Build history of the part. All positions in model axes, mm. Face numbers are marked on the shaded views. A direction names the side the tool comes from. Coordinates: 2 decimals unless noted, no trailing zeros. Order: outer loops, then holes, each group sorted by start corner. A loop starts at its lowest first (then second) coordinate and runs counter-clockwise, first axis right, second up. Notation, with made-up numbers: (55.25, 45) - (89.25, 45) arc R28 cw to (89.25, 67) - close; hole circle Ø9 at (6.5, -12). An arc over 180 degrees is marked (long way). Return JSON: item names as keys, results as strings.
Autodesk Inventor part; units mm, degrees
ref_plane "YZ Plane" through (0, 0, 0) normal (1, 0, 0) x (0, 1, 0)
ref_plane "XZ Plane" through (0, 0, 0) normal (0, 1, 0) x (-1, 0, 0)
ref_plane "XY Plane" through (0, 0, 0) normal (0, 0, 1) x (1, 0, 0)
sketch "Sketch2" plane through (0, 0, 0) normal (0, 1, 0) x (-1, 0, 0)
  line L0 (0, 0) -> (0, -39.2)
  line L1 (0, -39.2) -> (-69.3, -39.2)
  line L2 (-69.3, -39.2) -> (-69.3, 0)
  line L3 (-69.3, 0) -> (0, 0)
  dimension "d0" = 39.2
  dimension "d1" = 69.3
extrude "Extrusion1" add sketch "Sketch2" against normal blind 5
sketch "Sketch3" plane through (0, -5, 0) normal (0, -1, 0) x (1, 0, 0)
  line L0 (0, 0) -> (0, -39.2)
  line L1 (0, -39.2) -> (0, -34.2)
  line L2 (0, -34.2) -> (69.3, -34.2)
  line L3 (69.3, -39.2) -> (69.3, 0)
  line L4 (69.3, -39.2) -> (69.3, -34.2)
  line L5 (0, -39.2) -> (69.3, -39.2)
  dimension "d4" = 5
extrude "Extrusion2" add sketch "Sketch3" along normal blind 20
sketch "Sketch4" plane through (0, -5, -34.2) normal (0, 0, 1) x (1, 0, 0)
  line L0 (0, 5) -> (0, -20)
  line L1 (0, -20) -> (0, -18)
  line L2 (0, -18) -> (69.3, -18)
  line L3 (69.3, 5) -> (69.3, -20)
  line L4 (69.3, -20) -> (69.3, -18)
  line L5 (0, -20) -> (69.3, -20)
  line L6 (0, -20) -> (69.3, -20)
  dimension "d7" = 2
extrude "Extrusion3" add sketch "Sketch4" along normal blind 5
sketch "Sketch5" plane through (69.3, 0, 0) normal (1, 0, 0) x (0, 0, -1)
  line L0 (39.2, -25) -> (29.2, -25)
  line L1 (29.2, -25) -> (29.2, 0)
  line L2 (39.2, 0) -> (0, 0)
  line L3 (29.2, 0) -> (39.2, 0)
  line L4 (39.2, 0) -> (39.2, -25)
  line L5 (39.2, -25) -> (29.2, -25)
extrude "Extrusion4" add sketch "Sketch5" along normal blind 5
sketch "Sketch6" plane through (69.3, -5, 0) normal (1, 0, 0) x (0, 0, -1)
  line L0 (0, 5) -> (0, 0)
  line L1 (29.2, 0) -> (29.2, 5)
  line L2 (0, 5) -> (29.2, 5)
  line L3 (29.2, 5) -> (29.2, 0)
  line L4 (0, 0) -> (34.2, 0)
  line L5 (29.2, 0) -> (0, 0)
  line L6 (0, 0) -> (0, 5)
extrude "Extrusion5" add sketch "Sketch6" along normal blind 5
sketch "Sketch7" plane through (0, -5, -29.2) normal (0, 0, 1) x (1, 0, 0)
  line L0 (0, -20) -> (74.3, -20)
  line L1 (74.3, -20) -> (74.3, 0)
  line L2 (74.3, 0) -> (69.3, 0)
  line L3 (74.3, 0) -> (69.3, 0)
  line L4 (69.3, 0) -> (69.3, -18)
  line L5 (69.3, 0) -> (69.3, -20)
  line L6 (74.3, -20) -> (69.3, -20)
  point P0 (0, 5)
extrude "Extrusion6" add sketch "Sketch7" along normal up to surface (29.2 mm away)
sketch "Sketch8" plane through (0, 0, -39.2) normal (-1, 0, 0) x (0, 0, 1)
  line L0 (10, -25) -> (39.2, -25)
  line L1 (10, -25) -> (10, 0)
  line L2 (0, 0) -> (39.2, 0)
  line L3 (0, 0) -> (10, 0)
  line L4 (0, 0) -> (0, -25)
  line L5 (0, -25) -> (10, -25)
extrude "Extrusion7" add sketch "Sketch8" along normal blind 5
sketch "Sketch9" plane through (0, -5, 0) normal (-1, 0, 0) x (0, 0, 1)
  line L0 (-29.2, 5) -> (0, 5)
  line L1 (0, 5) -> (-29.2, 5)
  line L2 (-39.2, -20) -> (-29.2, -20)
  line L3 (-29.2, 5) -> (-29.2, -20)
  line L4 (0, 5) -> (0, -20)
  line L5 (-29.2, -20) -> (0, -20)
  line L6 (0, -20) -> (0, 5)
extrude "Extrusion8" add sketch "Sketch9" along normal blind 5
sketch "Sketch10" plane through (74.3, 0, 0) normal (1, 0, 0) x (0, 0, -1)
  line L0 (0, 0) -> (0, -25)
  line L1 (0, 0) -> (0, -3)
  line L2 (0, -3) -> (39.2, -3)
  line L3 (39.2, 0) -> (39.2, -25)
  line L4 (39.2, 0) -> (0, 0)
  line L5 (39.2, 0) -> (0, 0)
  line L6 (39.2, -3) -> (39.2, 0)
  dimension "d20" = 3
sketch "Sketch11" plane through (-5, 0, -39.2) normal (-1, 0, 0) x (0, 0, 1)
  line L0 (39.2, 0) -> (39.2, -25)
  line L1 (39.2, 0) -> (39.2, -3)
  line L2 (39.2, -3) -> (0, -3)
  line L3 (0, 0) -> (0, -25)
  line L4 (0, 0) -> (0, -3)
  line L5 (0, 0) -> (39.2, 0)
  dimension "d21" = 3
extrude "Extrusion9" add sketch "Sketch11" along normal blind 6
extrude "Extrusion10" add sketch "Sketch10" along normal blind 6
sketch "Sketch13" plane through (0, -5, 0) normal (0, -1, 0) x (1, 0, 0)
  line L0 (0, -34.2) -> (69.3, -34.2)
  arc A0 (32.15, -24) -> (37.15, -24) centre (34.65, -24) ccw
  line L1 (32.15, -24) -> (32.15, 0)
  line L2 (37.15, -24) -> (37.15, 0)
  line L3 (0, 0) -> (69.3, 0)
  dimension "d34" = 5
  dimension "d56" = 24
  dimension "d57" = 24
extrude "Extrusion13" cut sketch "Sketch13" against normal through all
sketch "Sketch15" plane through (0, 0, -39.2) normal (1, 0, 0) x (0, 0, -1)
  line L0 (0, -25) -> (-39.2, -25)
  line L1 (-10, -23) -> (-10, -25)
  line L2 (-39.2, -25) -> (-10, -25)
  line L3 (-10, -25) -> (-10, -23)
  line L4 (-5, -5) -> (-5, -23)
  line L5 (-10, -23) -> (-5, -23)
  line L6 (-5, -23) -> (-5, -5)
  line L7 (-39.2, -5) -> (-5, -5)
  line L8 (-5, -5) -> (-39.2, -5)
  line L9 (-10, -25) -> (-39.2, -25)
  line L10 (-39.2, -5) -> (-39.2, -25)
  point P0 (-39.2, 0)
extrude "Extrusion15" add sketch "Sketch15" along normal blind 0.4
sketch "Sketch16" plane through (69.3, 0, 0) normal (-1, 0, 0) x (0, 0, 1)
  line L0 (-34.2, -5) -> (0, -5)
  line L1 (0, -5) -> (0, -25)
  line L2 (-29.2, -25) -> (-29.2, -23)
  line L3 (0, -25) -> (-29.2, -25)
  line L4 (-29.2, -25) -> (-29.2, -23)
  line L5 (-29.2, -23) -> (-34.2, -23)
  line L6 (-34.2, -5) -> (-34.2, -23)
  line L7 (-34.2, -23) -> (-34.2, -5)
  line L8 (-34.2, -5) -> (0, -5)
  point P0 (0, 0)
extrude "Extrusion16" add sketch "Sketch16" along normal blind 0.4
sketch "Sketch17" plane through (0.4, -23, -34.2) normal (0, 0, 1) x (1, 0, 0)
  line L0 (0, 0) -> (30, 0)
  line L1 (0, 0) -> (68.5, 0)
  line L2 (68.5, 0) -> (37.5, 0)
  line L3 (37.5, 0) -> (37.5, 3)
  line L4 (30, 0) -> (30, 3)
  line L5 (30, 3) -> (30.8, 3)
  line L6 (37.5, 3) -> (36.7, 3)
  line L7 (34.3, 8.5) -> (30.8, 8.5)
  line L8 (30.8, 8.5) -> (30.8, 3)
  line L9 (36.7, 3) -> (30.8, 3)
  arc A0 (34.3, 3) -> (34.3, 8.5) centre (34.3, 5.75) ccw
  point P0 (-0.4, 23)
  dimension "d46" = 30
  dimension "d47" = 31
  dimension "d48" = 3
  dimension "d49" = 0.8
  dimension "d50" = 0.8
  dimension "d59" = 3.5
  dimension "d60" = 3.5
  dimension "d61" = 5.5
extrude "Extrusion17" add sketch "Sketch17" along normal blind 3 contours L8 L7 A0 L9
sketch "Sketch18" plane through (-11, -3, 0) normal (0, 0, 1) x (1, 0, 0)
  line L0 (6, 0) -> (0, 0)
  line L1 (0, 3) -> (0, 0)
  line L2 (0, 0) -> (6, 0)
  line L3 (6, 0) -> (6, -22)
  line L4 (6, 0) -> (6, -22)
  line L5 (6, -22) -> (11, -22)
  line L6 (85.3, -22) -> (6, -22)
  line L7 (11.4, -2) -> (11.4, -22)
  line L8 (11.4, -2) -> (79.9, -2)
  line L9 (79.9, -20) -> (11.4, -20)
  line L10 (79.9, -2) -> (79.9, -22)
  line L11 (85.3, -22) -> (85.3, 0)
  line L12 (79.9, -22) -> (85.3, -22)
  line L13 (85.3, -22) -> (85.3, 0)
  line L14 (85.3, 0) -> (91.3, 0)
  line L15 (91.3, 0) -> (93.4951, 0)
  line L16 (85.3, 0) -> (91.3, 0)
  line L17 (91.3, 0) -> (91.3, 3)
  line L18 (91.3, 3) -> (0, 3)
  line L19 (11.4, -2) -> (79.9, -2)
  line L20 (11.4, -2) -> (11.4, -22)
  line L21 (11, -22) -> (11.4, -22)
  point P0 (11, 3)
extrude "Extrusion18" cut sketch "Sketch18" against normal blind 17 contours L0 L1 L18 L17 L14 L11 L6 L10 L8 L7 L5 L3
sketch "Sketch19" plane through (-11, -3, -39.2) normal (0, -1, 0) x (1, 0, 0)
  line L0 (0, 22.2) -> (0, 0)
  line L1 (0, 11.1) -> (6, 11.1)
  line L2 (6, 0) -> (6, 22.2)
  circle A0 centre (3, 3) radius 1.65
  circle A1 centre (3, 3) radius 1.65
  circle A2 centre (3, 3) radius 2.5
  circle A3 centre (3, 19.2) radius 1.65
  circle A4 centre (3, 19.2) radius 2.5
  circle A5 centre (88.3, 3) radius 1.65
  circle A6 centre (88.3, 3) radius 1.65
  circle A7 centre (88.3, 3) radius 2.5
  circle A8 centre (88.3, 19.2) radius 1.65
  circle A9 centre (88.3, 19.2) radius 2.5
  point P0 (11, 39.2)
  dimension "d64" = 5
  dimension "d65" = 5
extrude "Extrusion19" cut sketch "Sketch19" against normal through all contours A3 | A8
extrude "Extrusion20" cut sketch "Sketch19" against normal blind 1.5 contours A3 | A4 | A9
properties part number "bottomcameraholder_6_24_2021"
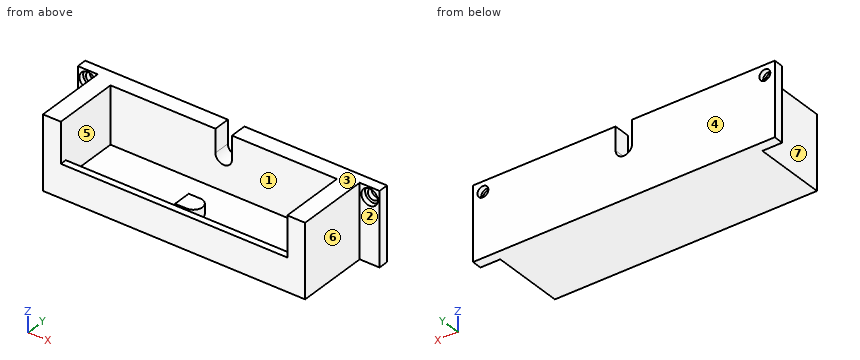
1. Mould opens along Y. For the marked faces 1, 2 and 3 say: pulls with the +Y half, pulls with the -Y half, needs draft (parallel to the pull), parting line crosses it, or undercut.
Check values:
{"face 1": "undercut", "face 2": "pulls with the -Y half", "face 3": "needs draft"}
2. Cut at D-D on z = -36. Give the cut face in (x, y).
Check values:
{"outline": "(-11, -3) - (-5, -3) - (-5, -25) - (74.3, -25) - (74.3, -3) - (80.3, -3) - (80.3, 0) - (-11, 0) - close"}
3. Drop flat-ended pins along their axis: pin 1 (5 mm diameter, centred on y = -19, z = -24, fed in from -X); pin 2 (2 mm diameter, centred on x = -8, z = -20, fed in from +Y); pin 3 (1.5 mm diameter, centred on x = 64.5, z = -20, fed in from -Y); pin 4 (1 mm diameter, centred on x = 32, y = -24, fed in from +Z). Give the stop position or say it passes through.
Check values:
{"pin 1": "x = -5", "pin 2": "through", "pin 3": "y = -5", "pin 4": "z = -29.2"}
4. Probe L1, parallel to Z at x = -8, y = -0.3; L2, parallel to X at y = -15.25, z = -24.5; L3, parallel to Z at x = 77.3, y = -2.1. List the from-to ranges inside material, lowest first.
Check values:
{"L1": "-39.2 to -21.65, -18.35 to -17", "L2": "-5 to 0.4, 68.9 to 74.3", "L3": "-39.2 to -22.5, -17.5 to -17"}
5. Cut at A-A on z = -20. State how many separate pieces and enclosed holes the cut face has, plus the area to 3 significant figures.
Check values:
{"separate pieces": "4", "enclosed holes": "0", "area": "599 mm²"}
6. Cut at C-C on y = -11.5. Give the cut face in (x, z).
Check values:
{"outline": "(-5, -39.2) - (74.3, -39.2) - (74.3, -17) - (68.9, -17) - (68.9, -34.2) - (0.4, -34.2) - (0.4, -17) - (-5, -17) - close"}
7. Cut at B-B on x = -8. Give the cut face in (y, z), plus the area to 4 significant figures.
Check values:
{"outline": "(-3, -39.2) - (0, -39.2) - (0, -21.65) - (-1.5, -21.65) - (-1.5, -22.5) - (-3, -22.5) - close; (-3, -17.5) - (-1.5, -17.5) - (-1.5, -18.35) - (0, -18.35) - (0, -17) - (-3, -17) - close", "area": "54.15 mm²"}
8. Tool access for the marked faces 4, 5, 6 and 7: list every direction of +Z, -Z, +X, -X, +Y, -Y with a clear straight run to the whole face (end or side of a thin tool).
Check values:
{"face 4": "+Z, -Z, +X, -X, +Y", "face 5": "+Z", "face 6": "+Z, -Z, +X, -Y", "face 7": "+Z, -Z, -X, -Y"}
